Work out the finished part from the listing and answer in its coordinate system (mm). A direction names the side the tool comes from. Give positions to 0.01 mm unless a question says otherwise; leave off trailing zeros. Order: outer loops, then holes, each group sorted by start corner. A loop starts at its lowest first (then second) coordinate and runs counter-clockwise, first axis right, second up. Notation, with made-up numbers: (-1, 4) -> (46, 4) arc R7 cw to (46, 10) -> close; hole circle Ø8 at (-10.75, 33). An arc over 180 degrees is marked (long way). Use a Markdown table: item, result. Add a question column.
```python
from build123d import *

# Parameters (mm, degrees)
CYLINDER115_R     = 1.6
CYLINDER115_DEPTH = 10
CYLINDER116_R     = 1.6
CYLINDER116_DEPTH = 10
CYLINDER117_R     = 1.6
CYLINDER117_DEPTH = 10
CYLINDER114_R     = 1.6
CYLINDER114_DEPTH = 10
BOX029_W          = 15
BOX029_H          = 15
BOX029_DEPTH      = 3
CYLINDER113_R     = 4
CYLINDER113_DEPTH = 15


with BuildPart() as cilindro115:
    # Cylinder115 → Cylinder115 (new body)
    with BuildSketch(Plane(origin=(32, 5, -20), x_dir=(1, 0, 0), z_dir=(0, 0, 1))):
        Circle(CYLINDER115_R)
    extrude(amount=CYLINDER115_DEPTH)


with BuildPart() as cilindro116:
    # Cylinder116 → Cylinder116 (new body)
    with BuildSketch(Plane(origin=(21, -6, -20), x_dir=(1, 0, 0), z_dir=(0, 0, 1))):
        Circle(CYLINDER116_R)
    extrude(amount=CYLINDER116_DEPTH)


with BuildPart() as cilindro117:
    # Cylinder117 → Cylinder117 (new body)
    with BuildSketch(Plane(origin=(21, 5, -20), x_dir=(1, 0, 0), z_dir=(0, 0, 1))):
        Circle(CYLINDER117_R)
    extrude(amount=CYLINDER117_DEPTH)


with BuildPart() as fusion058:
    # Cylinder114 → Cylinder114 (new body)
    with BuildSketch(Plane(origin=(32, -6, -20), x_dir=(1, 0, 0), z_dir=(0, 0, 1))):
        Circle(CYLINDER114_R)
    extrude(amount=CYLINDER114_DEPTH)

    # Fusion058: union Cilindro115, Cilindro116, Cilindro117
    add(cilindro115.part)
    add(cilindro116.part)
    add(cilindro117.part)


with BuildPart() as cubo028:
    # Box029 → Box029 (new body)
    with BuildSketch(Plane(origin=(-8, -8, 4), x_dir=(1, 0, 0), z_dir=(0, 0, 1))):
        with Locations((7.5, 7.5)):
            Rectangle(BOX029_W, BOX029_H)
    extrude(amount=BOX029_DEPTH)


with BuildPart() as esfera001:
    # Sphere001 → Sphere001 (revolve)
    with BuildSketch(Plane(origin=(0, 0, -16), x_dir=(1, 0, 0), z_dir=(0, -1, 0))):
        with BuildLine():
            ThreePointArc((0, -4), (4, 0), (0, 4))
            Line((0, 4), (0, -4))
        make_face()
    revolve(axis=Axis((0, 0, -16), (0, 0, 1)))


with BuildPart() as obj1:
    # Cylinder113 → Cylinder113 (new body)
    with BuildSketch(Plane.XY.offset(-15)):
        Circle(CYLINDER113_R)
    extrude(amount=CYLINDER113_DEPTH)

    # Fusion059: union Esfera001
    add(esfera001.part)


with BuildPart() as obj1_1:
    # Fusion059 placement: moved
    add(obj1.part.moved(Location((0, 0, 4))))

    # Fusion060: union Cubo028
    add(cubo028.part)


with BuildPart() as obj1_2:
    # Fusion060 placement: moved
    add(obj1_1.part.moved(Location((27, 0, -22))))

    # Cut019: cut Fusion058
    add(fusion058.part, mode=Mode.SUBTRACT)


with BuildPart() as obj1_3:
    # Cut019 placement: moved
    add(obj1_2.part.moved(Location((-81, 0.5, 0))))


solid = obj1_3.part
```
1) The part is cut by section A-A, the plane x = -60. Determine the outline of the cut face in (y, z).
2) Straight lines are drawn through the part: line 1 (Y direction, x = -49, z = -17.2); line 2 (X direction, y = 5.5, z = -16.75); line 3 (X direction, y = -6, z = -17). For each, find the intervals that lie inside material, in ascending order.
3) Which of the six approach directions +Z, -Z, +X, -X, +Y, -Y give full straight-line access (tool end or side, diameter ignored) to faces 1 (the cylindrical face through (-47.474, -5.019, -16.521)), 2 (the cylindrical face through (-50.185, 1.701, -25.605))?
4) The part is cut by section B-B, the plane y = 5.5. Determine the outline of the cut face in (x, z), then the cut area to 3 significant figures.
5) Determine the mould class of faces 3 (the cylindrical face through (-58.52, 4.89, -16.52)), 4 (the flat face through (-55, 0, -15)), 5 (the flat face through (-58, 2, -18)) for opening direction Z: released by +Z, released by -Z, zero draft, split by the parting line, or undercut.
6) Flat-ended cylindrical pins translate along their axes: pin 1 (3.5 mm diameter, centred on x = -49, y = 5.5, fed in from -Z); pin 2 (8 mm diameter, centred on y = 5, z = -21, fed in from +X); pin 3 (6 mm diameter, centred on x = -55.5, y = 4, fed in from -Z); pin 4 (3 mm diameter, centred on x = -60, y = -5.5, fed in from -Z). Find the tip coordinate at first contact, or state that the pin passes through.
7) The part is cut by section C-C, the plane x = -55.75. Determine the outline of the cut face in (y, z).
8) The part is cut by section D-D, the plane y = 0.5. Determine the outline of the cut face in (x, z), then the cut area to 3 significant figures.
A:
| question | item | result |
|---|---|---|
| 1 | outline | (-7.5, -18) -> (-7.1, -18) -> (-7.1, -15) -> (-7.5, -15) -> close; (-3.9, -18) -> (3.9, -18) -> (3.9, -15) -> (-3.9, -15) -> close; (7.1, -18) -> (7.5, -18) -> (7.5, -15) -> (7.1, -15) -> close |
| 2 | line 1 | -7.5 to -7.1, -3.9 to 3.9, 7.1 to 7.5 |
| 2 | line 2 | -62 to -61.6, -58.4 to -50.6, -47.4 to -47 |
| 2 | line 3 | -62 to -61.52, -58.48 to -50.52, -47.48 to -47 |
| 3 | face 1 | +Z, -Z |
| 3 | face 2 | -Z |
| 4 | outline | (-62, -18) -> (-61.6, -18) -> (-61.6, -15) -> (-62, -15) -> close; (-58.4, -18) -> (-50.6, -18) -> (-50.6, -15) -> (-58.4, -15) -> close; (-47.4, -18) -> (-47, -18) -> (-47, -15) -> (-47.4, -15) -> close |
| 4 | area | 25.8 mm^2 |
| 5 | face 3 | zero draft |
| 5 | face 4 | released by +Z |
| 5 | face 5 | released by -Z |
| 6 | pin 1 | z = -18 |
| 6 | pin 2 | x = -47 |
| 6 | pin 3 | z = -37.92 |
| 6 | pin 4 | through |
| 7 | outline | (-7.5, -18) -> (-3.1, -18) -> (-3.1, -33) -> (-2.96, -33) arc R3.6 ccw (long way) to (3.96, -33) -> (4.1, -33) -> (4.1, -18) -> (7.5, -18) -> (7.5, -15) -> (-7.5, -15) -> close |
| 8 | outline | (-62, -18) -> (-58, -18) -> (-58, -33) -> (-57.87, -33) arc R4 ccw (long way) to (-50.13, -33) -> (-50, -33) -> (-50, -18) -> (-47, -18) -> (-47, -15) -> (-62, -15) -> close |
| 8 | area | 198 mm^2 |
